For this review, take the finished solid that the model builds, in its own axes (mm). Face numbers are marked on the shaded views. A direction names the side the tool comes from. Round coordinates to 2 decimals unless told otherwise and drop trailing zeros. Order: outer loops, then holes, each group sorted by start corner. A loop starts at its lowest first (then second) coordinate and runs counter-clockwise, first axis right, second up. Notation, with made-up numbers: M 48.5,-5.75 L 83.5,-5.75 A7 cw 83.5,2.25 Z; hole C -3,85 d8. An arc over 180 degrees is marked long. Answer in a Markdown table with one row per item. Add a question column.
```python
from build123d import *

# Parameters (mm, degrees)
EXTRUDE1_DEPTH     = 9
SKETCH2_R          = 2.75
CUT_EXTRUDE1_DEPTH = 4
SKETCH3_R          = 2.75
CUT_EXTRUDE2_DEPTH = 4


with BuildPart() as part:
    # Sketch1 → Extrude1 (new body, symmetric)
    with BuildSketch(Plane.XY):
        with BuildLine():
            Line((0, 0), (0, 20))
            ThreePointArc((0, 20), (-2.121320344, 19.121320344), (-3, 17))
            Line((-3, 17), (-3, 5.25))
            ThreePointArc((-3, 5.25), (-3.659009742, 3.659009742), (-5.25, 3))
            Line((-5.25, 3), (-17, 3))
            ThreePointArc((-17, 3), (-19.121320344, 2.121320344), (-20, 0))
            Line((-20, 0), (0, 0))
        make_face()
    extrude(amount=EXTRUDE1_DEPTH, both=True)

    # Sketch2 → Cut-Extrude1 (cut, through all)
    with BuildSketch(Plane(origin=(0, 3, 0), x_dir=(1, 0, 0), z_dir=(0, 1, 0))):
        with Locations((-10, 0)):
            Circle(SKETCH2_R)
    extrude(amount=-CUT_EXTRUDE1_DEPTH, mode=Mode.SUBTRACT)

    # Sketch3 → Cut-Extrude2 (cut, through all)
    with BuildSketch(Plane.ZY.offset(3)):
        with Locations((0, 10)):
            Circle(SKETCH3_R)
    extrude(amount=-CUT_EXTRUDE2_DEPTH, mode=Mode.SUBTRACT)


solid = part.part
```
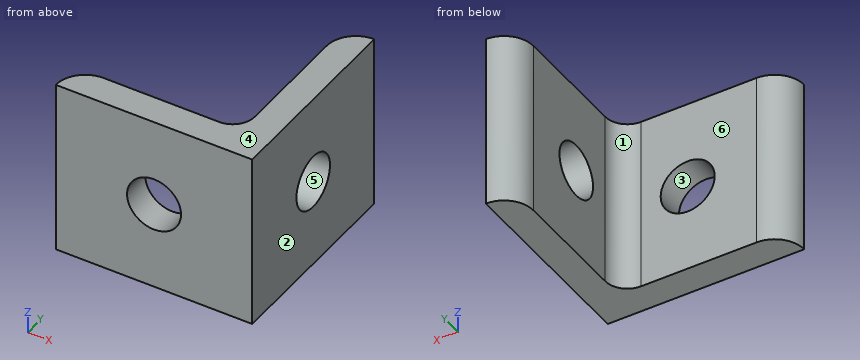
1. Consider section B-B on y = 10. Write out the cut boundary in (x, z).
2. For the marked faces 5 and 6, list the 3-axis set-ups (+Z, -Z, +X, -X, +Y, -Y) from which the entire face can be reached by the end or side of a thin tool; tool diameter is ignored.
3. Consider section D-D on z = 5.75. Write out the cut boundary in (x, y), plus the area to 3 significant figures.
4. Consider section A-A on z = 0. Write out the cut boundary in (x, y).
5. Consider section C-C on x = -10. Write out the cut boundary in (y, z).
6. The part is to be moulded in two halves that separate along X. For the marked faces 1, 2, 3 and 4, say which applies: pulls with the +X half, pulls with the -X half, needs draft (parallel to the pull), parting line crosses it, or undercut.
7. Clearance check with flat-ended pins moving along their axes: pin 1 Ø9 at (x, z) = (-10, 0) entering from +Y; pin 2 Ø3 at (y, z) = (3.5, -2) entering from -X; pin 3 Ø6 at (y, z) = (9, 3.5) entering from -X; pin 4 Ø6 at (x, y) = (-14, 7) entering from +Z. State where each tip first meets the part, or that it passes through.
8. To check wall thickness, follow probe 1 along Z at (x, y) = (-10, 1.3); probe 2 along Y at (x, z) = (-16.25, 5.75); probe 3 along X at (y, z) = (11.5, 7.75). State the ranges of each line that lie inside material, in increasing order. Write a range as [from, to].
Solved:
| question | item | result |
|---|---|---|
| 1 | outline | M -3,-9 L 0,-9 L 0,-2.75 L -3,-2.75 Z; M -3,2.75 L 0,2.75 L 0,9 L -3,9 Z |
| 2 | face 5 | +X, -X |
| 2 | face 6 | +Z, -Z, -X, +Y |
| 3 | outline | M -20,0 L 0,0 L 0,20 A3 ccw -3,17 L -3,5.25 A2.25 cw -5.25,3 L -17,3 A3 ccw Z |
| 3 | area | 108 mm^2 |
| 4 | outline | M -20,0 L -12.75,0 L -12.75,3 L -17,3 A3 ccw Z; M -7.25,0 L 0,0 L 0,7.25 L -3,7.25 L -3,5.25 A2.25 cw -5.25,3 L -7.25,3 Z; M -3,12.75 L 0,12.75 L 0,20 A3 ccw -3,17 Z |
| 5 | outline | M 0,-9 L 3,-9 L 3,-2.75 L 0,-2.75 Z; M 0,2.75 L 3,2.75 L 3,9 L 0,9 Z |
| 6 | face 1 | pulls with the -X half |
| 6 | face 2 | pulls with the +X half |
| 6 | face 3 | undercut |
| 6 | face 4 | needs draft |
| 7 | pin 1 | stops at y = 3 |
| 7 | pin 2 | stops at x = -19.24 |
| 7 | pin 3 | stops at x = -3 |
| 7 | pin 4 | passes through |
| 8 | probe 1 | z = [-9, -2.75], [2.75, 9] |
| 8 | probe 2 | y = [0, 3] |
| 8 | probe 3 | x = [-3, 0] |
